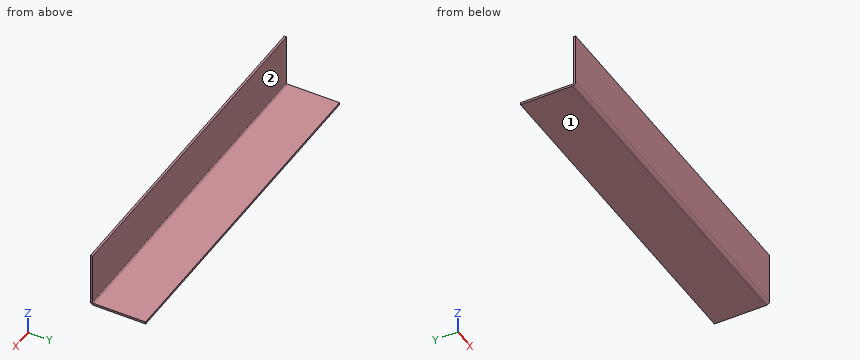
from build123d import *

# Parameters (mm, degrees)
SKETCH1_W                    = 250
SKETCH1_H                    = 1.5875
BASE_FLANGE1_DEPTH           = 40
EDGE_FLANGE1_STRIP_W         = 7.8232
EDGE_FLANGE1_STRIP_H         = 1.5875
EDGE_FLANGE1_STRIP_CUT_DEPTH = 250
EDGE_FLANGE1_DEPTH           = 250


# Sheet-metal steps are written as plain solids
with BuildPart() as part:
    # Sketch1 → Base-Flange1 (new body)
    with BuildSketch(Plane.XY):
        with Locations((0, -0.79375)):
            Rectangle(SKETCH1_W, SKETCH1_H)
    extrude(amount=BASE_FLANGE1_DEPTH)

    # Edge-Flange1 strip (across the edge) → Edge-Flange1 strip cut (cut)
    with BuildSketch(Plane.ZY.offset(-125)):
        with Locations((-1.5875, -0.79375)):
            Rectangle(EDGE_FLANGE1_STRIP_W, EDGE_FLANGE1_STRIP_H)
    extrude(amount=EDGE_FLANGE1_STRIP_CUT_DEPTH, mode=Mode.SUBTRACT)

    # Edge-Flange1 section (across the edge) → Edge-Flange1 (add)
    with BuildSketch(Plane.ZY.offset(-125)):
        with BuildLine():
            Line((0, 0.7366), (0, 38.4125))
            Line((0, 38.4125), (1.5875, 38.4125))
            Line((1.5875, 38.4125), (1.5875, 0.7366))
            ThreePointArc((1.5875, 0.7366), (1.803245145, 0.215745145), (2.3241, 0))
            Line((2.3241, 0), (2.3241, -1.5875))
            ThreePointArc((2.3241, -1.5875), (0.68071313, -0.90678687), (0, 0.7366))
        make_face()
    extrude(amount=EDGE_FLANGE1_DEPTH)


solid = part.part
Work out the finished part from the listing and answer in its coordinate system (mm). Face numbers are marked on the shaded views. A direction names the side the tool comes from. Give positions to 0.01 mm unless a question says otherwise; leave off trailing zeros. Order: outer loops, then holes, each group sorted by start corner. A loop starts at its lowest first (then second) coordinate and runs counter-clockwise, first axis right, second up. Notation, with made-up numbers: (20.25, -11) -> (46.25, -11) arc R21 ccw to (46.25, 11) -> close; hole circle Ø8 at (85, 15). An arc over 180 degrees is marked (long way). Answer as a JSON object with one key per item and string values. Group by question number.
1. Section A-A on x = -94 is taken. Determine the outline of the cut face in (y, z), plus the area to 3 significant figures.
2. Flat-ended cylindrical pins translate along their axes: pin 1 Ø3 at (x, y) = (46.5, 7.5) entering from +Z; pin 2 Ø3 at (x, z) = (14.5, 18) entering from +Y. Find the tip coordinate at first contact, or state that the pin passes through.
3. Section B-B on y = 10 is taken. Determine the outline of the cut face in (x, z), plus the area to 3 significant figures.
4. A tool of negligible diameter and unlimited length cuts with its end or side. For the marked faces 1 and 2, from which of +Z, -Z, +X, -X, +Y, -Y can it reach the whole face along a straight path? Write none if from no direction.
5. Consider line 1 along Y through (x, z) = (45, 12.5); line 2 along Z through (x, y) = (-26, 24). Determine where each line is inside the solid, lowest interval first. Write a range as [from, to].
6. Section C-C on z = 23 is taken. Determine the outline of the cut face in (x, y), plus the area to 3 significant figures.
Result sheet:
{
 "1": {"outline": "(-1.59, 2.32) arc R2.32 ccw to (0.74, 0) -> (38.41, 0) -> (38.41, 1.59) -> (0.74, 1.59) arc R0.74 cw to (0, 2.32) -> (0, 40) -> (-1.59, 40) -> close", "area": "123 mm^2"},
 "2": {"pin 1": "stops at z = 1.59", "pin 2": "stops at y = 0"},
 "3": {"outline": "(-125, 0) -> (125, 0) -> (125, 1.59) -> (-125, 1.59) -> close", "area": "397 mm^2"},
 "4": {"face 1": "-Z, +X, -X, +Y, -Y", "face 2": "+Z, +X, -X, +Y"},
 "5": {"line 1": "y = [-1.59, 0]", "line 2": "z = [0, 1.59]"},
 "6": {"outline": "(-125, -1.59) -> (125, -1.59) -> (125, 0) -> (-125, 0) -> close", "area": "397 mm^2"}
}
